Design review of the part built by this model. Coordinates are the model's own, in mm. Give positions to 0.01 mm unless a question says otherwise; leave off trailing zeros. Write each loop counter-clockwise with the first axis right and the second up, starting at its lowest first coordinate (ties: lowest second). Pieces come first, ordered by that corner, then holes. Notation, with made-up numbers: (4.5, -8.5) -> (16.5, -8.5) arc R28 cw to (16.5, 26.5) -> close; hole circle Ø5 at (40, -33). An arc over 180 degrees is marked (long way). Put each result on its own line as item: value. Start each with the question number.
from build123d import *

# Parameters (mm, degrees)
F2_R     = 27.5
F3_DEPTH = 20


# Not quite as in the source:
# - a feature names something its author has since deleted; it is built from what else it names


with BuildPart() as f1:
    # F0 (on Front) → F1 (revolve)
    with BuildSketch(Plane.XZ):
        with BuildLine():
            Line((0, -90), (0, 90))
            ThreePointArc((0, 90), (-90, 0), (0, -90))
        make_face()
    revolve(axis=Axis((0, 0, 3.2690457241), (0, 0, -1)))

    # F2 (on Front) → F3 (join)
    with BuildSketch(Plane.XZ):
        with Locations((-66.8500438333, 73.4359920025)):
            Circle(F2_R)
        with Locations((66.8500438333, 73.4359920025)):
            Circle(F2_R)
    extrude(amount=F3_DEPTH)

    # F4 (on face) → F5 (revolve)
    with BuildSketch(Plane(origin=(0, 0, 0), x_dir=(-1, 0, 0), z_dir=(0, 1, 0))):
        with BuildLine():
            Line((66.8500438333, 100.9359920025), (66.8500438333, 45.9359920025))
            ThreePointArc((66.8500438333, 45.9359920025), (94.3500438333, 73.4359920025), (66.8500438333, 100.9359920025))
        make_face()
    revolve(axis=Axis((-66.8500438333, 0, 71.019994095), (0, 0, -1)))

    # F6 (on face) → F7 (revolve)
    with BuildSketch(Plane(origin=(0, 0, 0), x_dir=(-1, 0, 0), z_dir=(0, 1, 0))):
        with BuildLine():
            Line((-66.8500438333, 100.9359920025), (-66.8500438333, 45.9359920025))
            ThreePointArc((-66.8500438333, 45.9359920025), (-39.3500438333, 73.4359920025), (-66.8500438333, 100.9359920025))
        make_face()
    revolve(axis=Axis((66.8500438333, 0, 79.5244728215), (0, 0, -1)))

    # F8 (on Right) → F9 (revolve)
    with BuildSketch(Plane.YZ):
        with BuildLine():
            ThreePointArc((0, -326.6847895979), (100.2179567321, -268.9169130562), (100.4595458508, -153.2419025898))
            ThreePointArc((100.4595458508, -153.2419025898), (65.487785005, -92.9832219274), (0, -69.2033424707))
            Line((0, -69.2033424707), (0, -326.6847895979))
        make_face()
    revolve(axis=Axis((0, 0, -34.6016712354), (0, 0, -1)))


solid = f1.part
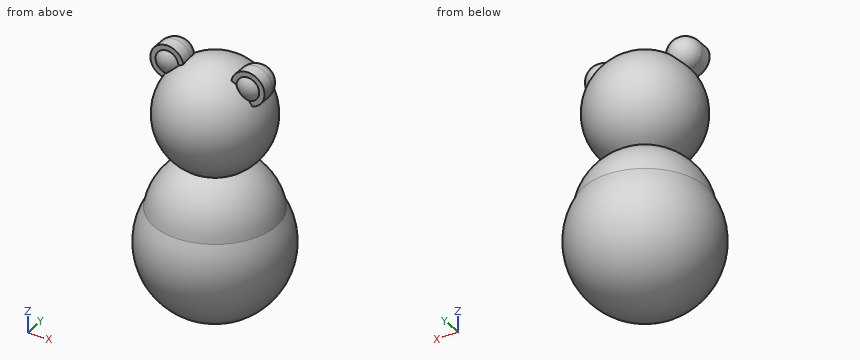
Q1. For pin 1 (3 mm diameter, centred on x = 0.5, z = -140, fed in from -Y); pin 2 (6 mm diameter, centred on y = -51, z = -124.5, fed in from +X); pin 3 (4 mm diameter, centred on x = -68.5, z = -242, fed in from -Y), all flat-tipped, find the tip position at first contact; note any pin that passes through.
Q2. Take a section at C-C on x = -13. Give the boundary of the cut face in (y, z).
Q3. Take a section at B-B on y = -80. Give the boundary of the cut face in (x, z).
Q4. Take a section at D-D on z = -130. Give the boundary of the cut face in (x, y), then the cut area to 3 significant figures.
Q5. Take a section at A-A on y = -14.5. Give the boundary of the cut face in (x, z), then the cut area to 3 significant figures.
Q6. To check wall thickness, follow probe 1 along Z at (x, y) = (50, 58.5); probe 2 along Z at (x, y) = (20, 65.5); probe 3 along X at (y, z) = (2, -2.5). State the ranges of each line that lie inside material, in increasing order. Write a range as from..to.
Result:
1. pin 1: stops at y = -97.63
1. pin 2: stops at x = 77.69
1. pin 3: stops at y = -89.71
2. outline: (-99.61, -153.24) arc R115.08 ccw (long way) to (99.61, -153.24) arc R101.23 ccw to (41.36, -78.87) arc R89.06 ccw (long way) to (-41.36, -78.87) arc R101.23 ccw to start
3. outline: (-60.76, -153.24) arc R83.74 ccw (long way) to (60.76, -153.24) arc R63.38 ccw to start; circle Ø82.46 at (0, 0)
4. outline: circle Ø186.7 at (0, 0)
4. area: 27,400 mm^2
5. outline: (-99.41, -153.24) arc R114.9 ccw (long way) to (99.41, -153.24) arc R101.03 ccw to (40.86, -78.87) arc R88.82 ccw to (75.22, 47.24) arc R27.5 ccw (long way) to (39.99, 79.32) arc R88.82 ccw to (-39.99, 79.32) arc R27.5 ccw (long way) to (-75.22, 47.24) arc R88.82 ccw to (-40.86, -78.87) arc R101.03 ccw to start
5. area: 73,200 mm^2
6. probe 1: z = -297.42..-104.22, -46.67..46.67
6. probe 2: z = -304.27..-95.59, -58.39..58.39
6. probe 3: x = -89.94..89.94
